Can you work these out from the model? Positions are in its coordinate system, mm. Face numbers are marked on the shaded views. A direction names the side the tool comes from. Coordinates: 2 decimals unless noted, no trailing zeros. Order: outer loops, then holes, each group sorted by start corner. A loop starts at its lowest first (then second) coordinate and runs counter-clockwise, first axis right, second up. Notation, with made-up numbers: (65, 80) -> (104, 80) arc R13 cw to (104, 91) -> close; hole circle Ø10 at (7, 89.25). An arc over 180 degrees is marked (long way). Write item = value, one per line.
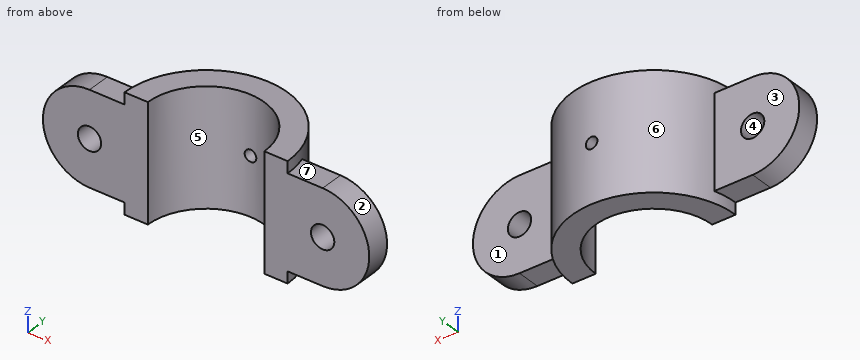
```python
from build123d import *

# Parameters (mm, degrees)
SLOTSKETCH_R      = 6.35
SLOTEXTRUDE_DEPTH = 12.7
ARCEXTRUDE_DEPTH  = 31.75
CENTERDRILL_D     = 6.35
ARCPROFILE_DEPTH  = 64.5000001


with BuildPart() as part:
    # slotSketch → slotExtrude (new body)
    with BuildSketch(Plane(origin=(0, 0, 0), x_dir=(1, 0, 0), z_dir=(0, 1, 0))):
        with BuildLine():
            Line((-63.5, 25.4), (63.5, 25.4))
            ThreePointArc((63.5, 25.4), (88.9, 0), (63.5, -25.4))
            Line((63.5, -25.4), (-63.5, -25.4))
            ThreePointArc((-63.5, -25.4), (-88.9, 0), (-63.5, 25.4))
        make_face()
        with Locations(Location((63.5, 0, 0), (0, 0, 270))):  # turned: the seam where the file's is
            Circle(SLOTSKETCH_R, mode=Mode.SUBTRACT)
        with Locations(Location((-63.5, 0, 0), (0, 0, 90))):  # turned: the seam where the file's is
            Circle(SLOTSKETCH_R, mode=Mode.SUBTRACT)
    extrude(amount=SLOTEXTRUDE_DEPTH)

    # Sketch3 → arcExtrude (add, symmetric)
    with BuildSketch(Plane.XY):
        with BuildLine():
            Line((-44.45, 0), (44.45, 0))
            ThreePointArc((44.45, 0), (0, 44.45), (-44.45, 0))
        make_face()
    extrude(amount=ARCEXTRUDE_DEPTH, both=True)

    # centerDrill (through all)
    with Locations(Plane(origin=(0, 0, 0), x_dir=(-1, 0, 0), z_dir=(0, -1, 0))):
        with Locations((0, 0)):
            Hole(CENTERDRILL_D / 2)

    # Sketch7 → arcProfile (cut, through all)
    with BuildSketch(Plane.XY.offset(31.75)):
        with BuildLine():
            Line((-31.75, 0), (31.75, 0))
            ThreePointArc((31.75, 0), (0, 31.75), (-31.75, 0))
        make_face()
    extrude(amount=-ARCPROFILE_DEPTH, mode=Mode.SUBTRACT)


solid = part.part
```
Item 1: For the marked faces 1, 2 and 3, which set-ups out of +Z, -Z, +X, -X, +Y, -Y let a thin tool reach every point of the face, with its end or its side?
A:
face_1 = +Z, -Z, +X, +Y
face_2 = +X, +Y, -Y
face_3 = +Z, -Z, -X, +Y
Item 2: I want a section at D-D, the plane y = 17.5. Please give me the cut outline in (x, z).
A:
outline = (-40.86, -31.75) -> (-26.49, -31.75) -> (-26.49, 31.75) -> (-40.86, 31.75) -> close; (26.49, -31.75) -> (40.86, -31.75) -> (40.86, 31.75) -> (26.49, 31.75) -> close
Item 3: I want a section at C-C, the plane z = 0. Please give me the cut outline in (x, y) (3 decimals), plus the area to 3 significant figures.
A:
outline = (-88.9, 0) -> (-69.85, 0) -> (-69.85, 12.7) -> (-88.9, 12.7) -> close; (-57.15, 0) -> (-31.75, 0) arc R31.75 cw to (-3.175, 31.591) -> (-3.175, 44.336) arc R44.45 ccw to (-42.597, 12.7) -> (-57.15, 12.7) -> close; (3.175, 31.591) arc R31.75 cw to (31.75, 0) -> (57.15, 0) -> (57.15, 12.7) -> (42.597, 12.7) arc R44.45 ccw to (3.175, 44.336) -> close; (69.85, 0) -> (88.9, 0) -> (88.9, 12.7) -> (69.85, 12.7) -> close
area = 2,260 mm2
Item 4: If I drill on probe 1 along Z at (x, y) = (0, 38) (3 decimals); probe 2 along Z at (x, y) = (63, 8); probe 3 along X at (y, z) = (4, 0), over which ranges is the centre line in solid material (lowest first)?
A:
probe_1 = -31.75 to -3.175, 3.175 to 31.75
probe_2 = -25.4 to -6.33, 6.33 to 25.4
probe_3 = -88.9 to -69.85, -57.15 to -31.5, 31.5 to 57.15, 69.85 to 88.9
Item 5: I want a section at A-A, the plane x = 0. Please give me the cut outline in (y, z) (3 decimals).
A:
outline = (31.75, -31.75) -> (44.45, -31.75) -> (44.45, -3.175) -> (31.75, -3.175) -> close; (31.75, 3.175) -> (44.45, 3.175) -> (44.45, 31.75) -> (31.75, 31.75) -> close
Item 6: I want a section at B-B, the plane y = 9.5. Please give me the cut outline in (x, z).
A:
outline = (-63.5, -25.4) -> (-43.42, -25.4) -> (-43.42, -31.75) -> (-30.3, -31.75) -> (-30.3, 31.75) -> (-43.42, 31.75) -> (-43.42, 25.4) -> (-63.5, 25.4) arc R25.4 ccw to start; (30.3, -31.75) -> (43.42, -31.75) -> (43.42, -25.4) -> (63.5, -25.4) arc R25.4 ccw to (63.5, 25.4) -> (43.42, 25.4) -> (43.42, 31.75) -> (30.3, 31.75) -> close; hole circle Ø12.7 at (-63.5, 0); hole circle Ø12.7 at (63.5, 0)
Item 7: If we mould it in two halves opening along X, with no side actions, what happens to the marked faces 4, 5, 6 and 7? For each: pulls with the +X half, pulls with the -X half, needs draft (parallel to the pull), parting line crosses it, or undercut.
A:
face_4 = undercut
face_5 = undercut
face_6 = parting line crosses it
face_7 = needs draft
Item 8: I'm going to push flat-ended pins straight in: P1, Ø1.5, axis at y = 22, z = 25, coming from the -X side; P2, Ø7.5, axis at x = 0, z = 0, coming from the -Y side; P3, Ø6.5, axis at x = 52.5, y = 6.5, coming from the +Z side; P4, Ø14, axis at x = 50.5, y = 3, coming from the -Z side. Where does each tip first touch, or does it pass through?
A:
P1 = -39.04
P2 = 31.53
P3 = 25.4
P4 = -31.75
